Work out the finished part from the listing and answer in its coordinate system (mm). Round coordinates to 2 decimals unless told otherwise and drop trailing zeros. Order: outer loops, then holes, each group sorted by start corner. A loop starts at its lowest first (then second) coordinate and runs counter-clockwise, first axis right, second up. Notation, with made-up numbers: (89.5, -9) - (125.5, -9) arc R19 ccw to (125.5, 0) - close; hole circle Ø10 at (-9, -34). An arc over 180 degrees is marked (long way). Answer in a Markdown table with one row per item.
from build123d import *

# Parameters (mm, degrees)
ESQUISSE1_R             = 37.5
ESQUISSE1_R_2           = 15
ESQUISSE1_R_3           = 23.5
BOSS_EXTRU_2_DEPTH      = 10
ESQUISSE2_W             = 10
ESQUISSE2_H             = 90
ENL_V_MAT_EXTRU_1_DEPTH = 10


with BuildPart() as part:
    # Esquisse1 → Boss.-Extru.2 (new body)
    with BuildSketch(Plane(origin=(0, 0, 0), x_dir=(1, 0, 0), z_dir=(0, 1, 0))):
        with BuildLine():
            Line((20, 480), (20, 60))
            ThreePointArc((20, 60), (64.470857294, 2.044450423), (131.961524227, 30))
            add(Edge.make_bspline(
                [(131.961524227, 30), (204.728797974, 156.036615257), (519.671151051, 149.91974963), (520, 150)],
                knots=[0, 0, 0, 0, 1, 1, 1, 1], degree=3))
            ThreePointArc((520, 150), (555.355339059, 164.644660941), (570, 200))
            Line((570, 200), (570, 340))
            ThreePointArc((570, 340), (555.355339059, 375.355339059), (520, 390))
            add(Edge.make_bspline(
                [(131.961524227, 510), (204.728797974, 383.963384743), (519.671151051, 390.08025037), (520, 390)],
                knots=[0, 0, 0, 0, 1, 1, 1, 1], degree=3))
            ThreePointArc((131.961524227, 510), (64.470857294, 537.955549577), (20, 480))
        make_face()
        with Locations(Location((405, 270, 0), (0, 0, 270))):
            Circle(ESQUISSE1_R, mode=Mode.SUBTRACT)
        with Locations(Location((520, 200, 0), (0, 0, 270))):
            Circle(ESQUISSE1_R_2, mode=Mode.SUBTRACT)
        with Locations(Location((520, 340, 0), (0, 0, 270))):
            Circle(ESQUISSE1_R_2, mode=Mode.SUBTRACT)
        with Locations(Location((80, 480, 0), (0, 0, 270))):
            Circle(ESQUISSE1_R_2, mode=Mode.SUBTRACT)
        with Locations(Location((80, 60, 0), (0, 0, 270))):
            Circle(ESQUISSE1_R_2, mode=Mode.SUBTRACT)
        with Locations(Location((175, 340, 0), (0, 0, 270))):
            Circle(ESQUISSE1_R_3, mode=Mode.SUBTRACT)
        with Locations(Location((175, 200, 0), (0, 0, 270))):
            Circle(ESQUISSE1_R_3, mode=Mode.SUBTRACT)
    extrude(amount=BOSS_EXTRU_2_DEPTH)

    # Esquisse2 → Enlèv. mat.-Extru.1 (cut)
    with BuildSketch(Plane(origin=(0, 10, 0), x_dir=(1, 0, 0), z_dir=(0, 1, 0))):
        with Locations((40, 175)):
            Rectangle(ESQUISSE2_W, ESQUISSE2_H)
        with Locations((40, 365)):
            Rectangle(ESQUISSE2_W, ESQUISSE2_H)
    extrude(amount=-ENL_V_MAT_EXTRU_1_DEPTH, mode=Mode.SUBTRACT)


solid = part.part
1) Each of these flat-tipped pins is pushed along its axis until it touches: pin 1 (24 mm diameter, centred on x = 80, z = -60, fed in from +Y); pin 2 (5 mm diameter, centred on x = 41, y = 6, fed in from +Z); pin 3 (1 mm diameter, centred on y = 8.5, z = -465, fed in from +X); pin 4 (3 mm diameter, centred on y = 3, z = -192.5, fed in from +X). Where does it stop, or does it pass through?
Filled in:
| item | result |
|---|---|
| pin 1 | passes through |
| pin 2 | stops at z = -12.38 |
| pin 3 | stops at x = 175.17 |
| pin 4 | stops at x = 569.64 |
2) The mould has two halves that part along Z. Classify faces 1 (the face through (63.41, 4.93, -2.34)), 2 (the face through (198.3, 4.93, -203.06)), 3 (the face through (555.742, 4.93, -374.964)), 4 (the face through (65.357, 4.93, -63.252)): released by +Z, released by -Z, zero draft, split by the parting line, or undercut.
Filled in:
| item | result |
|---|---|
| face 1 | released by +Z |
| face 2 | undercut |
| face 3 | released by -Z |
| face 4 | undercut |
3) Find the intervals of material crossed by probe 1 along X at (y, z) = (5.25, -200); probe 2 along Z at (x, y) = (43.5, 1.75); probe 3 along Z at (x, y) = (187, 7), in increasing order. Write a range as from..to.
Filled in:
| item | result |
|---|---|
| probe 1 | x = 20..35, 45..151.5, 198.5..505, 535..570 |
| probe 2 | z = -527.62..-410, -320..-220, -130..-12.38 |
| probe 3 | z = -456.7..-360.21, -319.79..-220.21, -179.79..-83.3 |
4) Find section A-A, the plane x = 80. Give the vertices of the cut face in (y, z).
Filled in:
| item | result |
|---|---|
| outline | (0, -540) - (10, -540) - (10, -495) - (0, -495) - close; (0, -465) - (10, -465) - (10, -75) - (0, -75) - close; (0, -45) - (10, -45) - (10, 0) - (0, 0) - close |
5) Find section B-B, the plane y = 8.25. Give the number of separate pieces and of enclosed holes in the cut face, then the cut area to 3 significant figures.
Filled in:
| item | result |
|---|---|
| separate pieces | 1 |
| enclosed holes | 9 |
| area | 172,000 mm^2 |
